Here's how the part is built. I have some questions about the finished solid (model axes, mm). A direction names the side the tool comes from. Coordinates: 2 decimals unless noted, no trailing zeros. Order: outer loops, then holes, each group sorted by start corner. A loop starts at its lowest first (then second) coordinate and runs counter-clockwise, first axis right, second up. Notation, with made-up numbers: (75, 55.25) - (108, 55.25) arc R34 ccw to (108, 85.25) - close; hole circle Ø9 at (-31.5, -11). An arc over 180 degrees is marked (long way). Answer in a Markdown table with one row per item. Add a question column.
Item 1: I want a section at C-C (y = 6.5). Please give me the cut outline in (x, z), plus the area to 3 significant figures.
Item 2: Thinking about a two-plate mould opening in X: for faces 4 (the cylindrical face through (-1.873, -11.226, 0.082)), 5 (the flat face through (0, -13, 0)), 6 (the cylindrical face through (26.5, 8.13, -27.07)), 7 (the cylindrical face through (-24.96, 6.41, 25.5)), which applies, +X half, -X half, draft (parallel to the pull), parting line (faces both ways), or undercut?
Item 3: I want a section at A-A (x = -15). Please give me the cut outline in (y, z), plus the area to 3 significant figures.
Item 4: On a 3-axis mill with a long thin cutter (end or side, diameter ignored), from which of +Z, -Z, +X, -X, +Y, -Y can I reach the whole of each face in a straight line? I mean faces 1 (the flat face through (7, 0, -7)), 2 (the cylindrical face through (-26.5, 5.18, 27.07)), 3 (the flat face through (-25.8, 6, 18)). Say none if no direction works.
Item 5: Will these pins go through, and if not, where does the flat tip stop? pin 1 Ø12 at (x, z) = (-13.5, -18.5) entering from -Y; pin 2 Ø8 at (y, z) = (-8.5, -2.5) entering from +X; pin 3 Ø1.1 at (x, z) = (-21, -23.5) entering from -Y.
Item 6: If I drill on line 1 along Z through (x, y) = (1.5, 9); line 2 along X through (y, z) = (6.5, 21.5); line 3 along Y through (x, z) = (16.5, -9.5), over which ranges is the centre line in solid material (lowest first)? Write a range as from..to.
Item 7: I want a section at D-D (y = 13.25). Please give me the cut outline in (x, z), plus the area to 3 significant figures.
Item 8: I want a section at B-B (z = 21). Please give me the cut outline in (x, y), plus the area to 3 significant figures.
```python
from build123d import *

# Parameters (mm, degrees)
EXTRUDE_1_DEPTH     = 16.5
SKETCH_2_W          = 56
SKETCH_2_H          = 17
CUT_EXTRUDE_1_DEPTH = 6
CUT_EXTRUDE_2_DEPTH = 8.3
SKETCH_4_R          = 7
SKETCH_4_R_2        = 0.5
EXTRUDE_2_DEPTH     = 1
SKETCH_5_R          = 4
EXTRUDE_3_DEPTH     = 4.5
SKETCH_6_R          = 2.8
EXTRUDE_4_DEPTH     = 4
SKETCH_7_R          = 1.875
EXTRUDE_5_DEPTH     = 3.5


with BuildPart() as part:
    # 草图1 → 凸台-拉伸1 (new body)
    with BuildSketch(Plane(origin=(0, 0, 0), x_dir=(1, 0, 0), z_dir=(0, 1, 0))):
        with BuildLine():
            Line((-23, 28.5), (23, 28.5))
            ThreePointArc((23, 28.5), (26.535533906, 27.035533906), (28, 23.5))
            Line((28, 23.5), (28, -23.5))
            ThreePointArc((28, -23.5), (26.535533906, -27.035533906), (23, -28.5))
            Line((23, -28.5), (-23, -28.5))
            ThreePointArc((-23, -28.5), (-26.535533906, -27.035533906), (-28, -23.5))
            Line((-28, -23.5), (-28, 23.5))
            ThreePointArc((-28, 23.5), (-26.535533906, 27.035533906), (-23, 28.5))
        make_face()
    extrude(amount=EXTRUDE_1_DEPTH)

    # 草图2 → 切除-拉伸1 (cut)
    with BuildSketch(Plane(origin=(0, 16.5, 0), x_dir=(1, 0, 0), z_dir=(0, 1, 0))):
        with Locations((0, -20)):
            Rectangle(SKETCH_2_W, SKETCH_2_H)
    extrude(amount=-CUT_EXTRUDE_1_DEPTH, mode=Mode.SUBTRACT)

    # 草图3 → 切除-拉伸2 (cut)
    with BuildSketch(Plane(origin=(0, 10.5, 0), x_dir=(1, 0, 0), z_dir=(0, 1, 0))):
        with BuildLine():
            Line((-25.8, -11.5), (25.8, -11.5))
            Line((25.8, -11.5), (25.8, -23.5))
            ThreePointArc((25.8, -23.5), (24.979898987, -25.479898987), (23, -26.3))
            Line((23, -26.3), (-23, -26.3))
            ThreePointArc((-23, -26.3), (-24.979898987, -25.479898987), (-25.8, -23.5))
            Line((-25.8, -23.5), (-25.8, -11.5))
        make_face()
    extrude(amount=-CUT_EXTRUDE_2_DEPTH, mode=Mode.SUBTRACT)

    # 草图4 → 凸台-拉伸2 (add)
    with BuildSketch(Plane.XZ):
        Circle(SKETCH_4_R)
        with Locations((-21, 23.5)):
            Circle(SKETCH_4_R_2)
        with Locations((21, 23.5)):
            Circle(SKETCH_4_R_2)
        with Locations((-21, -23.5)):
            Circle(SKETCH_4_R_2)
        with Locations((21, -23.5)):
            Circle(SKETCH_4_R_2)
    extrude(amount=EXTRUDE_2_DEPTH)

    # 草图5 → 凸台-拉伸3 (add)
    with BuildSketch(Plane.XZ.offset(1)):
        Circle(SKETCH_5_R)
    extrude(amount=EXTRUDE_3_DEPTH)

    # 草图6 → 凸台-拉伸4 (add)
    with BuildSketch(Plane.XZ.offset(5.5)):
        Circle(SKETCH_6_R)
    extrude(amount=EXTRUDE_4_DEPTH)

    # 草图7 → 凸台-拉伸5 (add)
    with BuildSketch(Plane.XZ.offset(9.5)):
        Circle(SKETCH_7_R)
    extrude(amount=EXTRUDE_5_DEPTH)


solid = part.part
```
Values follow:
| question | item | result |
|---|---|---|
| 1 | outline | (-28, -23.5) arc R5 ccw to (-23, -28.5) - (23, -28.5) arc R5 ccw to (28, -23.5) - (28, 23.5) arc R5 ccw to (23, 28.5) - (-23, 28.5) arc R5 ccw to (-28, 23.5) - close; hole (-25.8, 11.5) - (25.8, 11.5) - (25.8, 23.5) arc R2.8 ccw to (23, 26.3) - (-23, 26.3) arc R2.8 ccw to (-25.8, 23.5) - close |
| 1 | area | 2,410 mm^2 |
| 2 | face 4 | parting line |
| 2 | face 5 | draft |
| 2 | face 6 | +X half |
| 2 | face 7 | undercut |
| 3 | outline | (0, -28.5) - (16.5, -28.5) - (16.5, 11.5) - (2.2, 11.5) - (2.2, 26.3) - (10.5, 26.3) - (10.5, 28.5) - (0, 28.5) - close |
| 3 | area | 716 mm^2 |
| 4 | face 1 | -Y |
| 4 | face 2 | +Z, -X, +Y, -Y |
| 4 | face 3 | +Y |
| 5 | pin 1 | stops at y = 0 |
| 5 | pin 2 | stops at x = 4 |
| 5 | pin 3 | stops at y = -1 |
| 6 | line 1 | z = -28.5..11.5, 26.3..28.5 |
| 6 | line 2 | x = -28..-25.8, 25.8..28 |
| 6 | line 3 | y = 0..16.5 |
| 7 | outline | (-28, -23.5) arc R5 ccw to (-23, -28.5) - (23, -28.5) arc R5 ccw to (28, -23.5) - (28, 11.5) - (-28, 11.5) - close |
| 7 | area | 2,230 mm^2 |
| 8 | outline | (-28, 0) - (28, 0) - (28, 10.5) - (25.8, 10.5) - (25.8, 2.2) - (-25.8, 2.2) - (-25.8, 10.5) - (-28, 10.5) - close |
| 8 | area | 160 mm^2 |
